Read the model definition and answer for the solid it produces. Units are mm, in the model's axes. Give positions to 0.01 mm unless a question says otherwise; leave off trailing zeros. Write each loop counter-clockwise with the first axis right and the second up, starting at its lowest first coordinate (ties: lowest second). Pieces come first, ordered by that corner, then holes. Notation, with made-up numbers: M -38,31 L -20,31 A16 cw -20,57 Z; hole C 64,2.25 d6. An arc over 180 degrees is marked long. Put each result on its own line as item: value.
from build123d import *

# Parameters (mm, degrees)
SKETCH1_W           = 10
SKETCH1_H           = 10
SKETCH1_R           = 1.5875
BOSS_EXTRUDE1_DEPTH = 6


with BuildPart() as part:
    # Sketch1 → Boss-Extrude1 (new body)
    # profile 1 of 4: a face of its own
    with BuildSketch(Plane(origin=(0, 0, 0), x_dir=(1, 0, 0), z_dir=(0, 1, 0))):
        with BuildLine():
            Line((0, -5), (0, 5))
            Line((0, 5), (-5, 2.5))
            Line((-5, 2.5), (-5, 1.5875))
            ThreePointArc((-5, 1.5875), (-3.877467985, 1.122532015), (-3.4125, 0))
            ThreePointArc((-3.4125, 0), (-3.877467985, -1.122532015), (-5, -1.5875))
            Line((-5, -1.5875), (-5, -5))
            Line((-5, -5), (0, -5))
        make_face()
    # profile 2 of 4: a face of its own
    with BuildSketch(Plane(origin=(0, 0, 0), x_dir=(1, 0, 0), z_dir=(0, 1, 0))):
        with BuildLine():
            Line((-5, 2.5), (-10, 0))
            Line((-10, 0), (-10, -5))
            Line((-10, -5), (-5, -5))
            Line((-5, -5), (-5, -1.5875))
            ThreePointArc((-5, -1.5875), (-6.5875, 0), (-5, 1.5875))
            Line((-5, 1.5875), (-5, 2.5))
        make_face()
    # profile 3 of 4: a face of its own
    with BuildSketch(Plane(origin=(0, 0, 0), x_dir=(1, 0, 0), z_dir=(0, 1, 0))):
        Polygon((0, 5), (-10, 5), (-10, 0), (-5, 2.5), align=None)
    # profile 4 of 4: a face of its own
    with BuildSketch(Plane(origin=(0, 0, 0), x_dir=(1, 0, 0), z_dir=(0, 1, 0))):
        with Locations((5, 0)):
            Rectangle(SKETCH1_W, SKETCH1_H)
        with Locations(Location((5, 0, 0), (0, 0, 270))):
            Circle(SKETCH1_R, mode=Mode.SUBTRACT)
    extrude(amount=BOSS_EXTRUDE1_DEPTH)


solid = part.part
(1) Section B-B on z = 0.25 is taken. Determine the outline of the cut face in (x, y).
Result:
outline: M -10,0 L -6.57,0 L -6.57,6 L -10,6 Z; M -3.43,0 L 3.43,0 L 3.43,6 L -3.43,6 Z; M 6.57,0 L 10,0 L 10,6 L 6.57,6 Z
(2) For a pull along Z with two mould halves and no side action, classify faces 1 (the face through (-10, 3, 0)), 2 (the face through (3.45, 2.96, -0.34)), 3 (the face through (0, 3, -5)) as +Z half, -Z half, draft (parallel to the pull), parting line (faces both ways), or undercut.
Result:
face 1: draft
face 2: undercut
face 3: -Z half
(3) Section A-A on x = 5 is taken. Determine the outline of the cut face in (y, z).
Result:
outline: M 0,-5 L 6,-5 L 6,-1.59 L 0,-1.59 Z; M 0,1.59 L 6,1.59 L 6,5 L 0,5 Z
(4) Given pin 1 Ø5 at (x, z) = (5, 0) entering from +Y, flat-ended and moving along its own axis, determine where the tip first touches the part or whether it passes through.
Result:
pin 1: stops at y = 6
(5) Section C-C on y = 4.05 is taken. Determine the outline of the cut face in (x, z) (1 decimal), and give its area (3 significant figures).
Result:
outline: M -10,-5 L 10,-5 L 10,5 L -10,5 Z; hole C -5,0 d3.2; hole C 5,0 d3.2
area: 184 mm²
(6) Straight lines are drawn through the part: line 1 along X through (y, z) = (3.5, 0); line 2 along X through (y, z) = (3.65, -0.75); line 3 along Z through (x, y) = (6, 4.6). For each, find the intervals that lie inside material, in ascending order. Write a range as from..to.
Result:
line 1: x = -10..-6.59, -3.41..3.41, 6.59..10
line 2: x = -10..-6.4, -3.6..3.6, 6.4..10
line 3: z = -5..-1.23, 1.23..5
